Check sheet for the modelled part. Datum: model origin and axes. Units: mm. A direction names the side the tool comes from. Coordinates: 2 decimals unless noted, no trailing zeros. Loops run counter-clockwise (first coordinate to the right, second up) from the corner with the lowest first, then second, coordinate; pieces in that order, holes last. Notation, with made-up numbers: (23.5, 25.5) -> (35.5, 25.5) arc R25 ccw to (35.5, 63.5) -> close; hole circle Ø9 at (-26.5, -28.75). An arc over 180 degrees is marked (long way). Use CSV: the item, a comma, the result in double quotes. Start each with the question number.
1. Sectioned sample at A-A, the plane z = 3. Record the cut outline in (x, y), and give its area (3 significant figures).
2. Sectioned sample at B-B, the plane x = 0. Record the cut outline in (y, z).
3. Gauge pin test, flat ends, axial feed: pin 1 (6 mm diameter, centred on x = 0, y = 80, fed in from +Z); pin 2 (2 mm diameter, centred on x = -1.5, y = 20.5, fed in from +Z); pin 3 (2 mm diameter, centred on x = -6.5, z = 4, fed in from +Y); pin 4 (2 mm diameter, centred on x = -3, z = 4, fed in from +Y). Record the tip position at first contact, or that the pin passes through.
4. Sectioned sample at C-C, the plane y = 1.5. Record the cut outline in (x, z).
5. Thickness scan on L1, parallel to Y at x = 0, z = 1.45; L2, parallel to Y at x = 0, z = 9.75; L3, parallel to X at y = 0, z = 5. Record the ranges inside material, lowest first.
6. Sectioned sample at D-D, the plane x = -8. Record the cut outline in (y, z), and give its area (3 significant figures).
7. Set-up check for faces 1 (the face through (-0.867, -3.905, 0.986)), 2 (the face through (3.645, 10.802, 4.028)): record each of +Z, -Z, +X, -X, +Y, -Y from which the full face is reachable in a straight line by a thin tool's end or side.
8. Release check for a two-part mould opening along Y. For faces 3 (the face through (-5, 82, 12)), 4 (the face through (-1.302, 89.915, 7.249)), 5 (the face through (2.376, 75.431, 5.916)), 6 (the face through (-3.616, 10.984, 4.028)) record: pulls with the +Y half, pulls with the -Y half, needs draft (parallel to the pull), parting line crosses it, or undercut.
```python
from build123d import *

# Parameters (mm, degrees)
SKETCH_1_R          = 4
EXTRUDE_1_DEPTH     = 6
SKETCH_1_3_R        = 10
SKETCH_1_3_R_2      = 5.15
EXTRUDE_2_DEPTH     = 12
CUT_EXTRUDE_1_DEPTH = 4


with BuildPart() as part:
    # Sketch 1 → Extrude 1 (new body)
    with BuildSketch(Plane.XY):
        with BuildLine():
            ThreePointArc((-10, 0), (0, -10), (10, 0))
            Line((10, 0), (10, 80))
            ThreePointArc((10, 80), (0, 70), (-10, 80))
            Line((-10, 80), (-10, 0))
        make_face()
        Circle(SKETCH_1_R, mode=Mode.SUBTRACT)
    extrude(amount=EXTRUDE_1_DEPTH)

    # Sketch 1_3 → Extrude 2 (add)
    with BuildSketch(Plane.XY):
        with Locations((0, 80)):
            Circle(SKETCH_1_3_R)
        with Locations((0, 80)):
            Circle(SKETCH_1_3_R_2, mode=Mode.SUBTRACT)
    extrude(amount=EXTRUDE_2_DEPTH)

    # Sketch 2 → Cut-Extrude 1 (cut)
    with BuildSketch(Plane.XY.offset(6)):
        with BuildLine():
            Line((-2.6, 17.4), (-4.661300265, 4.385462329))
            ThreePointArc((-4.661300265, 4.385462329), (0, -6.4), (4.661300265, 4.385462329))
            Line((4.661300265, 4.385462329), (2.6, 17.4))
            ThreePointArc((2.6, 17.4), (0, 20), (-2.6, 17.4))
        make_face()
    extrude(amount=-CUT_EXTRUDE_1_DEPTH, mode=Mode.SUBTRACT)


solid = part.part
```
Completed:
1,outline,"(-10, 0) arc R10 ccw to (10, 0) -> (10, 80) arc R10 ccw to (-10, 80) -> close; hole circle Ø10.3 at (0, 80); hole (-4.66, 4.39) arc R6.4 ccw (long way) to (4.66, 4.39) -> (2.6, 17.4) arc R2.6 ccw to (-2.6, 17.4) -> close"
1,area,"1,610 mm²"
2,outline,"(-10, 0) -> (-4, 0) -> (-4, 2) -> (-6.4, 2) -> (-6.4, 6) -> (-10, 6) -> close; (4, 0) -> (74.85, 0) -> (74.85, 12) -> (70, 12) -> (70, 6) -> (20, 6) -> (20, 2) -> (4, 2) -> close; (85.15, 0) -> (90, 0) -> (90, 12) -> (85.15, 12) -> close"
3,pin 1,"through"
3,pin 2,"z = 6"
3,pin 3,"y = 88.35"
3,pin 4,"y = 89.8"
4,outline,"(-10, 0) -> (-3.71, 0) -> (-3.71, 2) -> (-6.22, 2) -> (-6.22, 6) -> (-10, 6) -> close; (3.71, 0) -> (10, 0) -> (10, 6) -> (6.22, 6) -> (6.22, 2) -> (3.71, 2) -> close"
5,L1,"-10 to -4, 4 to 74.85, 85.15 to 90"
5,L2,"70 to 74.85, 85.15 to 90"
5,L3,"-10 to -6.4, 6.4 to 10"
6,outline,"(-6, 0) -> (86, 0) -> (86, 12) -> (74, 12) -> (74, 6) -> (-6, 6) -> close"
6,area,"624 mm²"
7,face 1,"+Z, -Z"
7,face 2,"+Z"
8,face 3,"needs draft"
8,face 4,"parting line crosses it"
8,face 5,"undercut"
8,face 6,"undercut"
